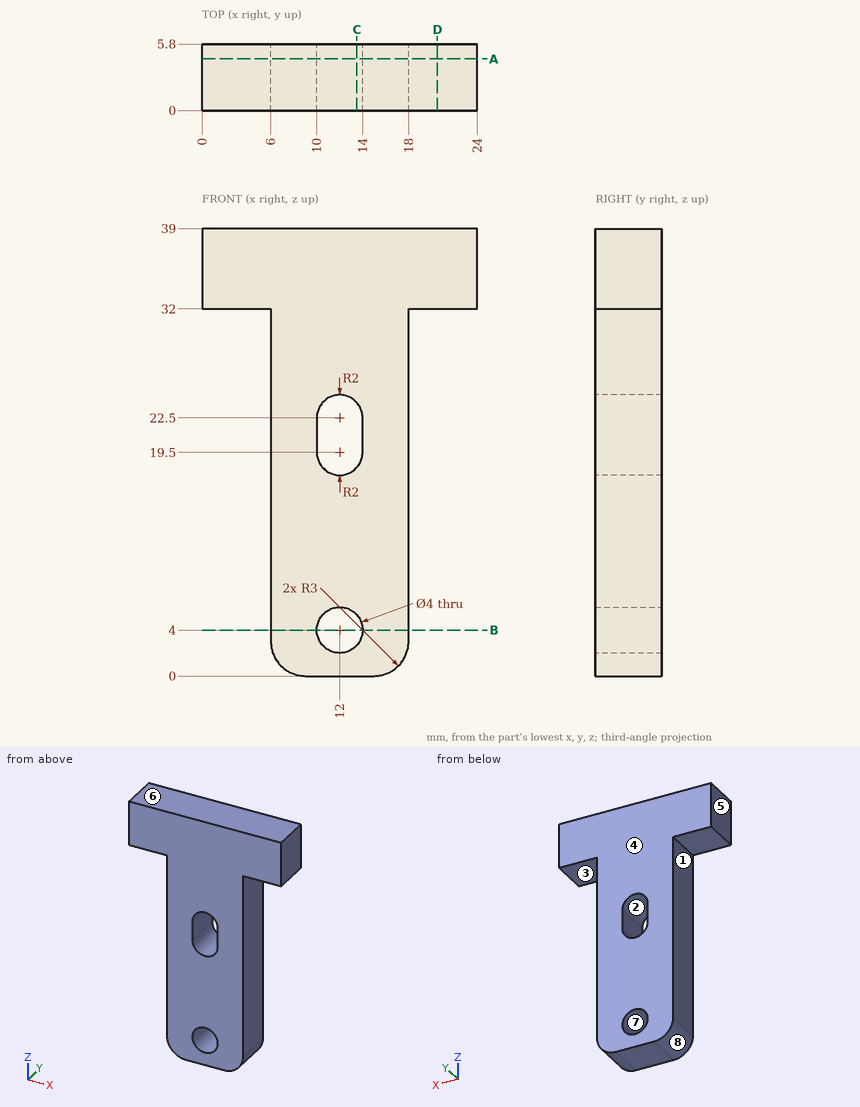
Verification items for this drawing (mm, ordinates from the low corner). A direction names the side the tool comes from. Round coordinates to 2 decimals unless told otherwise and drop trailing zeros. Write each loop counter-clockwise with the first axis right and the second up, starting at its lowest first coordinate (ties: lowest second). Pieces come first, ordered by that corner, then holes. Notation, with made-up numbers: (-31.5, 58) - (26.5, 58) arc R27 cw to (26.5, 79) - close; hole circle Ø5 at (-18.75, -15). An arc over 180 degrees is marked (long way). Answer as a JSON object with one key per item and string values. Group by question number.
Q1. Go/stop test with flat-tipped pins: pin 1 Ø1.5 at (y, z) = (3, 25) entering from -X; pin 2 Ø1.5 at (x, z) = (19.5, 18) entering from +Y; pin 3 Ø1.7 at (x, y) = (20, 3) entering from -Z; pin 4 Ø1.5 at (y, z) = (3, 21.5) entering from +X. Record where each tip stops, or that it passes through.
Q2. Thickness scan on line 1 (Z direction, x = 11.5, y = 1.55); line 2 (Z direction, x = 21.5, y = 4.05); line 3 (X direction, y = 1.65, z = 25). Record the ranges inside material, lowest first.
Q3. Tool access check on the marked faces 1, 2, 3, 4 and 5. Record the directions out of +Z, -Z, +X, -X, +Y, -Y that give a thin tool (end or side, any length) a straight path to the whole face; none if there is none.
Q4. Section check D-D, the plane x = 20.5. Enter the section's corners in (y, z), plus the area to 3 significant figures.
Q5. Section check B-B, the plane z = 4. Enter the section's corners in (x, y).
Q6. Section check A-A, the plane y = 4.5. Enter the section's corners in (x, z).
Q7. Mould release check, pull along Z, two halves, no side actions. Record for the marked faces 6, 7 and 8: released by +Z, released by -Z, zero draft, split by the parting line, or undercut.
Q8. Section check C-C, the plane x = 13.5. Enter the section's corners in (y, z), plus the area to 3 significant figures.
Found:
{
 "1": {"pin 1": "stops at x = 6", "pin 2": "passes through", "pin 3": "stops at z = 32", "pin 4": "stops at x = 18"},
 "2": {"line 1": "z = 0 to 2.06, 5.94 to 17.56, 24.44 to 39", "line 2": "z = 32 to 39", "line 3": "x = 6 to 18"},
 "3": {"face 1": "-Z, -X, +Y, -Y", "face 2": "+Y, -Y", "face 3": "-Z, +X, +Y, -Y", "face 4": "+Z, -Z, +X, -X, +Y", "face 5": "+Z, -Z, -X, +Y, -Y"},
 "4": {"outline": "(0, 32) - (5.8, 32) - (5.8, 39) - (0, 39) - close", "area": "40.6 mm^2"},
 "5": {"outline": "(6, 0) - (10, 0) - (10, 5.8) - (6, 5.8) - close; (14, 0) - (18, 0) - (18, 5.8) - (14, 5.8) - close"},
 "6": {"outline": "(0, 32) - (6, 32) - (6, 3) arc R3 ccw to (9, 0) - (15, 0) arc R3 ccw to (18, 3) - (18, 32) - (24, 32) - (24, 39) - (0, 39) - close; hole circle Ø4 at (12, 4); hole (10, 19.5) arc R2 ccw to (14, 19.5) - (14, 22.5) arc R2 ccw to (10, 22.5) - close"},
 "7": {"face 6": "released by +Z", "face 7": "undercut", "face 8": "released by -Z"},
 "8": {"outline": "(0, 0) - (5.8, 0) - (5.8, 2.68) - (0, 2.68) - close; (0, 5.32) - (5.8, 5.32) - (5.8, 18.18) - (0, 18.18) - close; (0, 23.82) - (5.8, 23.82) - (5.8, 39) - (0, 39) - close", "area": "178 mm^2"}
}
